```python
from build123d import *

# Parameters (mm, degrees)
MAIN_STOCK_START                   = -2.751909566
SKETCH_1_W                         = 57.95
SKETCH_1_H                         = 49.98
MAIN_STOCK_DEPTH                   = 5
SKETCH_3_R                         = 0.8
PCB_5XD1P6_M2_THROUGH_DEPTH        = 71.63982517
SKETCH_10_W                        = 7.5
SKETCH_10_H                        = 9.2
TYPEC_BOTTOM_RECESS_A_DEPTH        = 0.5
SKETCH_11_W                        = 9.2
SKETCH_11_H                        = 7.5
TYPEC_BOTTOM_RECESS_B_DEPTH        = 0.5
SKETCH_12_W                        = 62
SKETCH_12_H                        = 54
SKETCH_12_W_2                      = 49.91
SKETCH_12_H_2                      = 41.94
INSET_BASE_PERIMETER_DEPTH         = 5.1
SKETCH_13_R                        = 0.8
HORIZONTAL_BASE_M2_0_0_00028_DEPTH = 5
HORIZONTAL_BASE_M2_0_0_04963_START = -5
SKETCH_14_R                        = 0.8
HORIZONTAL_BASE_M2_0_0_04963_DEPTH = 5
SKETCH_15_R                        = 0.8
HORIZONTAL_BASE_M2_1_0_00028_DEPTH = 5
SKETCH_16_R                        = 0.8
HORIZONTAL_BASE_M2_1_0_04166_DEPTH = 5


with BuildPart() as part:
    # 草图1 → Main_Stock (new body)
    with BuildSketch(Plane.XY.offset(MAIN_STOCK_START)):
        with Locations((24.675, 20.69)):
            Rectangle(SKETCH_1_W, SKETCH_1_H)
    extrude(amount=MAIN_STOCK_DEPTH)

    # 草图3 → PCB_5xD1p6_M2_Through (cut, through all)
    with BuildSketch(Plane.XY.offset(2.248090434)):
        with Locations((23.428293927, 20.276755792)):
            Circle(SKETCH_3_R)
        with Locations((2.206251763, 39.333791606)):
            Circle(SKETCH_3_R)
        with Locations((47.653340917, 39.333791606)):
            Circle(SKETCH_3_R)
        with Locations((47.653340917, 1.976720232)):
            Circle(SKETCH_3_R)
        with Locations((2.206251763, 1.976720232)):
            Circle(SKETCH_3_R)
    extrude(amount=-PCB_5XD1P6_M2_THROUGH_DEPTH, mode=Mode.SUBTRACT)

    # 草图10 → TypeC_Bottom_Recess_A (cut)
    with BuildSketch(Plane.XY.offset(2.248090434)):
        with Locations((45.6, 31.7)):
            Rectangle(SKETCH_10_W, SKETCH_10_H)
    extrude(amount=-TYPEC_BOTTOM_RECESS_A_DEPTH, mode=Mode.SUBTRACT)

    # 草图11 → TypeC_Bottom_Recess_B (cut)
    with BuildSketch(Plane.XY.offset(2.248090434)):
        with Locations((33.523, 37.63)):
            Rectangle(SKETCH_11_W, SKETCH_11_H)
    extrude(amount=-TYPEC_BOTTOM_RECESS_B_DEPTH, mode=Mode.SUBTRACT)

    # 草图12 → Inset_Base_Perimeter (cut)
    with BuildSketch(Plane(origin=(0, 0, -2.751909566), x_dir=(-1, 0, 0), z_dir=(0, 0, -1))):
        with Locations((-25, 21)):
            Rectangle(SKETCH_12_W, SKETCH_12_H)
        with Locations((-24.675, 20.69)):
            Rectangle(SKETCH_12_W_2, SKETCH_12_H_2, mode=Mode.SUBTRACT)
    extrude(amount=-INSET_BASE_PERIMETER_DEPTH, mode=Mode.SUBTRACT)

    # 草图13 → Horizontal_Base_M2_0_-0.00028 (cut)
    with BuildSketch(Plane.ZY.offset(0.28)):
        with Locations((-0.75, 20)):
            Circle(SKETCH_13_R)
        with Locations((-0.75, 33)):
            Circle(SKETCH_13_R)
    extrude(amount=-HORIZONTAL_BASE_M2_0_0_00028_DEPTH, mode=Mode.SUBTRACT)

    # 草图14 → Horizontal_Base_M2_0_0.04963 (cut)
    with BuildSketch(Plane(origin=(49.63, 0, 0), x_dir=(0, 0, -1), z_dir=(1, 0, 0)).offset(HORIZONTAL_BASE_M2_0_0_04963_START)):
        with Locations(Location((0.75, 20, 0), (0, 0, 180))):
            Circle(SKETCH_14_R)
        with Locations((0.75, 24)):
            Circle(SKETCH_14_R)
    extrude(amount=HORIZONTAL_BASE_M2_0_0_04963_DEPTH, mode=Mode.SUBTRACT)

    # 草图15 → Horizontal_Base_M2_1_-0.00028 (cut)
    with BuildSketch(Plane.XZ.offset(0.28)):
        with Locations(Location((14.5, -0.75, 0), (0, 0, 270))):
            Circle(SKETCH_15_R)
        with Locations(Location((34.85, -0.75, 0), (0, 0, 270))):
            Circle(SKETCH_15_R)
    extrude(amount=-HORIZONTAL_BASE_M2_1_0_00028_DEPTH, mode=Mode.SUBTRACT)

    # 草图16 → Horizontal_Base_M2_1_0.04166 (cut)
    with BuildSketch(Plane(origin=(0, 41.66, 0), x_dir=(1, 0, 0), z_dir=(0, 1, 0))):
        with Locations(Location((5, 0.75, 0), (0, 0, 270))):
            Circle(SKETCH_16_R)
        with Locations(Location((45.2, 0.75, 0), (0, 0, 270))):
            Circle(SKETCH_16_R)
    extrude(amount=-HORIZONTAL_BASE_M2_1_0_04166_DEPTH, mode=Mode.SUBTRACT)


solid = part.part
```
For this review, take the finished solid that the model builds, in its own axes (mm). A direction names the side the tool comes from. Coordinates: 2 decimals unless noted, no trailing zeros. Loops run counter-clockwise (first coordinate to the right, second up) from the corner with the lowest first, then second, coordinate; pieces in that order, holes last.
1. Insertion check: P1, Ø0.8, axis at x = 14.5, z = -1, coming from the -Y side; P2, Ø0.5, axis at y = 20, z = -1, coming from the +X side; P3, Ø0.8, axis at y = 33, z = -0.5, coming from the -X side. Each pin has a flat end and moves straight along its axis. Give the tip position at first contact, or say it passes through.
2. Add section A-A, the plane x = 45.2. Give the boundary of the cut face in (y, z), then the cut area to 3 significant figures.
3. For line 1 (Y direction, x = 3.15, z = -0.75); line 2 (X direction, y = 38.2, z = -0.75); line 3 (Z direction, x = 34.85, y = 3.45), list the stretches that pass through material, from the lowest coordinate up.
4. Add section B-B, the plane y = 24. Give the boundary of the cut face in (x, z), then the cut area to 3 significant figures.
5. Mouldability with a two-part tool opening along X and no side actions: class faces 1 (the cylindrical face through (47.1, 20.71, -0.38)), 2 (the cylindrical face through (22.63, 20.31, -0.22)), 3 (the cylindrical face through (44.42, 39.19, -0.92)), 4 (the flat face through (44.63, 20, -1)) as +X half, -X half, draft (parallel to the pull), parting line (faces both ways), or undercut.
6. For faces 5 (the flat face through (35, 4.72, -1)), 6 (the flat face through (4.72, 20, -1)), 7 (the flat face through (46, 32, 1.748)), list the 3-axis set-ups (+Z, -Z, +X, -X, +Y, -Y) from which the entire face can be reached by the end or side of a thin tool; tool diameter is ignored.
7. Add section D-D, the plane z = -0.75. Count the separate pieces of the cut face and the enclosed holes in it, then the cut area to 3 significant figures.
8. Add section C-C, the plane x = 34.85. Give the boundary of the cut face in (y, z), then the cut area to 3 significant figures.
Result:
1. P1: stops at y = 4.72
1. P2: stops at x = 44.63
1. P3: stops at x = 4.72
2. outline: (-0.28, -2.75) - (41.66, -2.75) - (41.66, -1.55) - (36.66, -1.55) - (36.66, 0.05) - (41.66, 0.05) - (41.66, 2.25) - (36.3, 2.25) - (36.3, 1.75) - (27.1, 1.75) - (27.1, 2.25) - (-0.28, 2.25) - close; hole circle Ø1.6 at (20, -0.75); hole circle Ø1.6 at (24, -0.75)
2. area: 193 mm2
3. line 1: y = -0.28 to 19.2, 20.8 to 32.2, 33.8 to 41.66
3. line 2: x = -0.28 to 4.2, 5.8 to 44.4, 46 to 49.63
3. line 3: z = -2.75 to -1.55, 0.05 to 2.25
4. outline: (-0.28, -2.75) - (49.63, -2.75) - (49.63, -1.55) - (44.63, -1.55) - (44.63, 0.05) - (49.63, 0.05) - (49.63, 2.25) - (-0.28, 2.25) - close
4. area: 242 mm2
5. face 1: draft
5. face 2: undercut
5. face 3: undercut
5. face 4: +X half
6. face 5: -Y
6. face 6: -X
6. face 7: +Z
7. separate pieces: 1
7. enclosed holes: 5
7. area: 2,020 mm2
8. outline: (-0.28, -2.75) - (41.66, -2.75) - (41.66, 2.25) - (41.38, 2.25) - (41.38, 1.75) - (33.88, 1.75) - (33.88, 2.25) - (-0.28, 2.25) - (-0.28, 0.05) - (4.72, 0.05) - (4.72, -1.55) - (-0.28, -1.55) - close
8. area: 198 mm2
